```python
from build123d import *

# Parameters (mm, degrees)
SKETCH1_W               = 18
SKETCH1_H               = 15
BOSS_EXTRUDE1_DEPTH     = 8
SKETCH2_W               = 6
SKETCH2_H               = 2.5
SKETCH2_W_2             = 10
SKETCH2_H_2             = 2
CUT_EXTRUDE1_DEPTH      = 1
CUT_EXTRUDE1_DEPTH_BACK = 16
SKETCH4_W               = 5
SKETCH4_H               = 3.5
BOSS_EXTRUDE2_DEPTH     = 5
SKETCH5_W               = 35
SKETCH5_H               = 30
BOSS_EXTRUDE3_DEPTH     = 4
SKETCH6_R               = 1.905
CUT_EXTRUDE2_DEPTH      = 1
CUT_EXTRUDE2_DEPTH_BACK = 9


with BuildPart() as part:
    # Sketch1 → Boss-Extrude1 (new body)
    with BuildSketch(Plane(origin=(0, 0, 0), x_dir=(1, 0, 0), z_dir=(0, 1, 0))):
        with Locations((9, 7.5)):
            Rectangle(SKETCH1_W, SKETCH1_H)
    extrude(amount=BOSS_EXTRUDE1_DEPTH)

    # Sketch2 → Cut-Extrude1 (cut, two sides)
    with BuildSketch(Plane.XY) as cut_extrude1_sk:
        with Locations((9, 6.75)):
            Rectangle(SKETCH2_W, SKETCH2_H)
        with Locations((9, 4.5)):
            Rectangle(SKETCH2_W_2, SKETCH2_H_2)
    extrude(amount=CUT_EXTRUDE1_DEPTH, mode=Mode.SUBTRACT)
    extrude(cut_extrude1_sk.sketch, amount=-CUT_EXTRUDE1_DEPTH_BACK, mode=Mode.SUBTRACT)

    # Sketch4 → Boss-Extrude2 (add)
    with BuildSketch(Plane.XY):
        with Locations((9, 1.75)):
            Rectangle(SKETCH4_W, SKETCH4_H)
        Polygon((11.5, 3.5), (11.5, 0), (18, 0), (18, 8), (12, 8), (12, 5.5), (14, 5.5), (14, 3.5), align=None)
        Polygon((6, 8), (0, 8), (0, 0), (6.5, 0), (6.5, 3.5), (4, 3.5), (4, 5.5), (6, 5.5), align=None)
        Polygon((6.5, 8), (6, 8), (6, 5.5), (4, 5.5), (4, 3.5), (6.5, 3.5), align=None)
        Polygon((12, 8), (11.5, 8), (11.5, 3.5), (14, 3.5), (14, 5.5), (12, 5.5), align=None)
    extrude(amount=BOSS_EXTRUDE2_DEPTH)

    # Sketch5 → Boss-Extrude3 (add)
    with BuildSketch(Plane(origin=(0, 0, 0), x_dir=(-1, 0, 0), z_dir=(0, -1, 0))):
        with Locations((-9, 0)):
            Rectangle(SKETCH5_W, SKETCH5_H)
    extrude(amount=-BOSS_EXTRUDE3_DEPTH)

    # Sketch6 → Cut-Extrude2 (cut, two sides)
    with BuildSketch(Plane(origin=(0, 0, 0), x_dir=(-1, 0, 0), z_dir=(0, -1, 0))) as cut_extrude2_sk:
        with Locations((3.7, 2.3)):
            Circle(SKETCH6_R)
        with Locations((-21.7, -10.4)):
            Circle(SKETCH6_R)
        with Locations((3.7, -10.4)):
            Circle(SKETCH6_R)
        with Locations((-21.7, 2.3)):
            Circle(SKETCH6_R)
    extrude(amount=CUT_EXTRUDE2_DEPTH, mode=Mode.SUBTRACT)
    extrude(cut_extrude2_sk.sketch, amount=-CUT_EXTRUDE2_DEPTH_BACK, mode=Mode.SUBTRACT)


solid = part.part
```
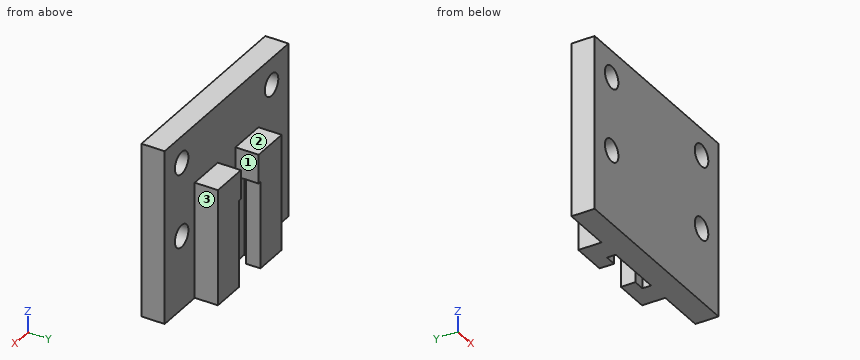
Geometry check sheet. Reference: the model listing, model coordinates, mm. Face numbers are marked on the shaded views. A direction names the side the tool comes from. Give positions to 0.01 mm unless a question says otherwise; leave off trailing zeros. Order: outer loops, then holes, each group sorted by start corner. A loop starts at its lowest first (then second) coordinate and runs counter-clockwise, first axis right, second up.
1. Access from +Z, -Z, +X, -X, +Y, -Y to the whole of each face (thin tool, end or side, straight path). Record for the marked faces 1, 2 and 3.
2. Section check C-C, the plane z = 10.4. Enter the section's corners in (x, y) (3 decimals).
3. Gauge pin test, flat ends, axial feed: pin 1 Ø2.5 at (x, z) = (21.7, 10.4) entering from -Y; pin 2 Ø2 at (y, z) = (5.5, -7.5) entering from +X; pin 3 Ø2 at (x, y) = (4.5, 7) entering from +Z; pin 4 Ø1 at (x, z) = (10, 1) entering from +Y. Record the tip position at first contact, or that the pin passes through.
4. Section check D-D, the plane y = 1.75. Enter the section's corners in (x, z) (3 decimals).
5. Section check A-A, the plane y = 4.5. Enter the section's corners in (x, z).
6. Section check B-B, the plane x = -3.7. Enter the section's corners in (y, z) (3 decimals).
7. Thickness scan on L1, parallel to Z at x = 21.7, y = 2.5 (3 decimals); L2, parallel to X at y = 1.3, z = -2.3 (3 decimals); L3, parallel to Y at x = 12.5, z = -12. Record the ranges inside material, lowest first.
Values follow:
1. face 1: +Z, -Z, +Y
1. face 2: +Z, +X, -X, +Y
1. face 3: +Z, -Z, +X, +Y
2. outline: (-8.5, 0) - (-5.605, 0) - (-5.605, 4) - (-8.5, 4) - close; (-1.795, 0) - (19.795, 0) - (19.795, 4) - (-1.795, 4) - close; (23.605, 0) - (26.5, 0) - (26.5, 4) - (23.605, 4) - close
3. pin 1: passes through
3. pin 2: stops at x = 18
3. pin 3: stops at z = 5
3. pin 4: stops at y = 4
4. outline: (-8.5, -15) - (26.5, -15) - (26.5, 15) - (-8.5, 15) - close; hole circle Ø3.81 at (-3.7, -2.3); hole circle Ø3.81 at (-3.7, 10.4); hole circle Ø3.81 at (21.7, -2.3); hole circle Ø3.81 at (21.7, 10.4)
5. outline: (0, -15) - (4, -15) - (4, 0) - (6.5, 0) - (6.5, 5) - (0, 5) - close; (11.5, 0) - (14, 0) - (14, -15) - (18, -15) - (18, 5) - (11.5, 5) - close
6. outline: (0, -15) - (4, -15) - (4, -4.205) - (0, -4.205) - close; (0, -0.395) - (4, -0.395) - (4, 8.495) - (0, 8.495) - close; (0, 12.305) - (4, 12.305) - (4, 15) - (0, 15) - close
7. L1: z = -15 to -4.205, -0.395 to 8.495, 12.305 to 15
7. L2: x = -8.5 to -5.605, -1.795 to 19.795, 23.605 to 26.5
7. L3: y = 0 to 4, 5.5 to 8
